from build123d import *

# Parameters (mm, degrees)
SKETCH_1_W          = 15
SKETCH_1_H          = 15
SKETCH_1_W_2        = 13
SKETCH_1_H_2        = 13
EXTRUDE_1_DEPTH     = 181.6
SKETCH_2_R          = 2.6
CUT_EXTRUDE_1_DEPTH = 183.372722741
SKETCH_3_R          = 2.1
CUT_EXTRUDE_2_DEPTH = 183.372722741


with BuildPart() as part:
    # ｽｹｯﾁ1 → 押し出し-薄板1 (new body)
    with BuildSketch(Plane.XY):
        Rectangle(SKETCH_1_W, SKETCH_1_H)
        Rectangle(SKETCH_1_W_2, SKETCH_1_H_2, mode=Mode.SUBTRACT)
    extrude(amount=EXTRUDE_1_DEPTH)

    # ｽｹｯﾁ2 → ｶｯﾄ - 押し出し1 (cut, through all)
    with BuildSketch(Plane(origin=(0, 7.5, 0), x_dir=(1, 0, 0), z_dir=(0, 1, 0))):
        with Locations(Location((0, -132.86, 0), (0, 0, 180))):
            Circle(SKETCH_2_R)
        with Locations(Location((0, -60.74, 0), (0, 0, 180))):
            Circle(SKETCH_2_R)
    extrude(amount=-CUT_EXTRUDE_1_DEPTH, mode=Mode.SUBTRACT)

    # ｽｹｯﾁ3 → ｶｯﾄ - 押し出し2 (cut, through all)
    with BuildSketch(Plane.ZY.offset(7.5)):
        with Locations(Location((174.1, 0, 0), (0, 0, 270))):
            Circle(SKETCH_3_R)
        with Locations(Location((146.6, 0, 0), (0, 0, 270))):
            Circle(SKETCH_3_R)
        with Locations(Location((35, 0, 0), (0, 0, 270))):
            Circle(SKETCH_3_R)
        with Locations(Location((7.5, 0, 0), (0, 0, 270))):
            Circle(SKETCH_3_R)
    extrude(amount=-CUT_EXTRUDE_2_DEPTH, mode=Mode.SUBTRACT)


solid = part.part
Could you check a few things on this model? Use its own coordinates, in mm. A direction names the side the tool comes from. Round coordinates to 2 decimals unless told otherwise and drop trailing zeros. Order: outer loops, then holes, each group sorted by start corner. A loop starts at its lowest first (then second) coordinate and runs counter-clockwise, first axis right, second up.
(1) Imagine slicing it at C-C (y = 3.75). Write out the boundary of the cut face in (x, z).
Response values:
outline: (-7.5, 0) - (-6.5, 0) - (-6.5, 181.6) - (-7.5, 181.6) - close; (6.5, 0) - (7.5, 0) - (7.5, 181.6) - (6.5, 181.6) - close
(2) Imagine slicing it at B-B (z = 35). Write out the boundary of the cut face in (x, y).
Response values:
outline: (-7.5, -7.5) - (7.5, -7.5) - (7.5, -2.1) - (6.5, -2.1) - (6.5, -6.5) - (-6.5, -6.5) - (-6.5, -2.1) - (-7.5, -2.1) - close; (-7.5, 2.1) - (-6.5, 2.1) - (-6.5, 6.5) - (6.5, 6.5) - (6.5, 2.1) - (7.5, 2.1) - (7.5, 7.5) - (-7.5, 7.5) - close
(3) Which directions (+Z, -Z, +X, -X, +Y, -Y) give clear straight access to the entire face, cutting with the end or side of a thin tool? Please do faces 4 (the cylindrical face through (-7, 0, 172)), 5 (the flat face through (-6.5, 0, 90)).
Response values:
face 4: +X, -X
face 5: +Z, -Z
(4) Imagine slicing it at A-A (x = 0). Write out the boundary of the cut face in (y, z).
Response values:
outline: (-7.5, 0) - (-6.5, 0) - (-6.5, 58.14) - (-7.5, 58.14) - close; (-7.5, 63.34) - (-6.5, 63.34) - (-6.5, 130.26) - (-7.5, 130.26) - close; (-7.5, 135.46) - (-6.5, 135.46) - (-6.5, 181.6) - (-7.5, 181.6) - close; (6.5, 0) - (7.5, 0) - (7.5, 58.14) - (6.5, 58.14) - close; (6.5, 63.34) - (7.5, 63.34) - (7.5, 130.26) - (6.5, 130.26) - close; (6.5, 135.46) - (7.5, 135.46) - (7.5, 181.6) - (6.5, 181.6) - close
(5) Imagine slicing it at D-D (z = 97). Write out the boundary of the cut face in (x, y).
Response values:
outline: (-7.5, -7.5) - (7.5, -7.5) - (7.5, 7.5) - (-7.5, 7.5) - close; hole (-6.5, -6.5) - (6.5, -6.5) - (6.5, 6.5) - (-6.5, 6.5) - close
(6) If we mould it in two halves opening along Y, with no side actions, what happens to faces 1 (the flat face through (0, 7.5, 90)), 2 (the cylindrical face through (0.56, 7.01, 58.2)), 3 (the flat face through (0, -6.5, 90))? For each: released by +Y, released by -Y, zero draft, split by the parting line, or undercut.
Response values:
face 1: released by +Y
face 2: zero draft
face 3: undercut
(7) Please list where these lines run through material, in increasing order: line 1 along Z through (x, y) = (7.1, 0); line 2 along X through (y, z) = (-2.25, 141).
Response values:
line 1: z = 0 to 5.4, 9.6 to 32.9, 37.1 to 144.5, 148.7 to 172, 176.2 to 181.6
line 2: x = -7.5 to -6.5, 6.5 to 7.5
(8) I'm going to push a flat-ended pin straight in: pin 1 (5.5 mm diameter, centred on y = 0, z = 35, fed in from -X). Where does the tip first touch, or does it pass through?
Response values:
pin 1: stops at x = -7.5
